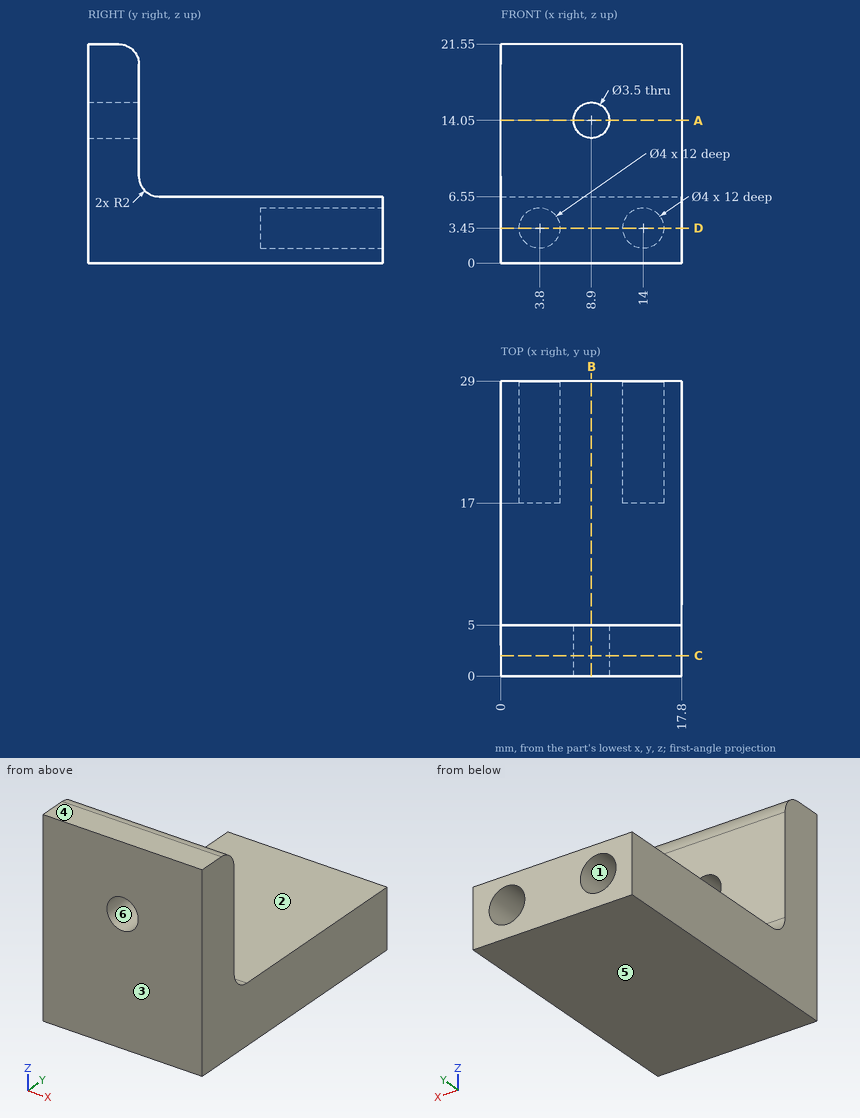
Part print with two shaded views. Sizes in mm from the minimum x, y, z corner. A direction names the side the tool comes from. Give positions to 0.01 mm unless a question says otherwise; leave off trailing zeros. Order: outer loops, then holes, each group sorted by start corner. A loop starts at its lowest first (then second) coordinate and runs counter-clockwise, first axis right, second up. Notation, with made-up numbers: M -39,7.25 L 14,7.25 A22 ccw 14,24.25 Z; hole C 19,21 d11. An arc over 180 degrees is marked long. Write item = value, one per line.
Q1. Cut at C-C, the plane y = 2. List the corners of the cut face in (x, z), then the cut area to 3 significant figures.
Derived:
outline = M 0,0 L 17.8,0 L 17.8,21.55 L 0,21.55 Z; hole C 8.9,14.05 d3.5
area = 374 mm2
Q2. Flat gauge pins, fed straight in: pin 1 (3.5 mm diameter, centred on x = 12.5, z = 16.5, fed in from +Y); pin 2 (2.5 mm diameter, centred on x = 14, z = 3.45, fed in from +Y); pin 3 (5.5 mm diameter, centred on x = 7.5, y = 14.5, fed in from +Z). Where does each tip first touch, or does it go through?
Derived:
pin_1 = 5
pin_2 = 17
pin_3 = 6.55
Q3. Cut at A-A, the plane z = 14.05. List the corners of the cut face in (x, y).
Derived:
outline = M 0,0 L 7.15,0 L 7.15,5 L 0,5 Z; M 10.65,0 L 17.8,0 L 17.8,5 L 10.65,5 Z
Q4. Drill centre lines: line 1 (X direction, y = 24.25, z = 3.45); line 2 (X direction, y = 1.45, z = 14.05); line 3 (Z direction, x = 3.8, y = 22). Where is each one in solid material? Low to high. Write a range as [from, to].
Derived:
line_1 = [0, 1.8], [5.8, 12], [16, 17.8]
line_2 = [0, 7.15], [10.65, 17.8]
line_3 = [0, 1.45], [5.45, 6.55]
Q5. Cut at B-B, the plane x = 8.9. List the corners of the cut face in (y, z), then the cut area to 3 significant figures.
Derived:
outline = M 0,0 L 29,0 L 29,6.55 L 7,6.55 A2 cw 5,8.55 L 5,12.3 L 0,12.3 Z; M 0,15.8 L 5,15.8 L 5,19.55 A2 ccw 3,21.55 L 0,21.55 Z
area = 247 mm2
Q6. Cut at D-D, the plane z = 3.45. List the corners of the cut face in (x, y).
Derived:
outline = M 0,0 L 17.8,0 L 17.8,29 L 16,29 L 16,17 L 12,17 L 12,29 L 5.8,29 L 5.8,17 L 1.8,17 L 1.8,29 L 0,29 Z
Q7. Tool access for the marked faces 1, 2 and 3: list every direction of +Z, -Z, +X, -X, +Y, -Y with a clear straight run to the whole face (end or side of a thin tool).
Derived:
face_1 = +Y
face_2 = +Z, +X, -X, +Y
face_3 = +Z, -Z, +X, -X, -Y
Q8. Two-plate mould, pull along Z, no slides. Class the marked faces 4, 5 and 6: pulls with the +Z half, pulls with the -Z half, needs draft (parallel to the pull), parting line crosses it, or undercut.
Derived:
face_4 = pulls with the +Z half
face_5 = pulls with the -Z half
face_6 = undercut
